Autodesk Inventor part; units mm, degrees
ref_plane "YZ Plane" through (0, 0, 0) normal (1, 0, 0) x (0, 1, 0)
ref_plane "XZ Plane" through (0, 0, 0) normal (0, 1, 0) x (-1, 0, 0)
ref_plane "XY Plane" through (0, 0, 0) normal (0, 0, 1) x (1, 0, 0)
sketch "Sketch1" plane through (0, 0, 0) normal (0, 1, 0) x (-1, 0, 0)
  line L0 (0, 0) -> (-101.6, 0)
  line L1 (-101.6, 0) -> (-101.6, -88.9)
  line L2 (-101.6, -88.9) -> (0, -88.9)
  line L3 (0, -88.9) -> (0, 0)
  line L4 (-50.8, -88.9) -> (-23.8125, -88.9)
  line L5 (-50.8, -88.9) -> (-77.7875, -88.9)
  line L6 (-77.7875, -88.9) -> (-77.7875, -82.55)
  line L7 (-23.8125, -88.9) -> (-23.8125, -82.55)
  circle A0 centre (-23.8125, -82.55) radius 1.905
  circle A1 centre (-77.7875, -82.55) radius 1.905
  dimension "d0" = 101.6
  dimension "d1" = 88.9
  dimension "d2" = 26.9875
  dimension "d3" = 26.9875
  dimension "d4" = 6.35
  dimension "d5" = 6.35
  dimension "d6" = 3.81
  dimension "d7" = 3.81
extrude "Extrusion1" add sketch "Sketch1" along normal blind 3.175
sketch "Sketch2" plane through (0, 0, 0) normal (0, -1, 0) x (1, 0, 0)
  line L0 (101.6, -88.9) -> (0, -88.9)
  line L1 (50.8, -88.9) -> (50.8, -12.7)
  line L2 (50.8, -12.7) -> (76.2, -12.7)
  line L3 (76.2, -12.7) -> (25.4, -12.7)
  line L4 (25.4, -12.7) -> (25.4, -6.35)
  line L5 (25.4, -6.35) -> (76.2, -6.35)
  line L6 (76.2, -6.35) -> (76.2, -12.7)
  point P0 (0, 0)
  dimension "d10" = 76.2
  dimension "d11" = 25.4
  dimension "d12" = 50.8
  dimension "d13" = 6.35
extrude "Extrusion2" add sketch "Sketch2" along normal blind 6.35
sketch "Sketch3" plane through (0, 3.175, 0) normal (0, 1, 0) x (1, 0, 0)
  line L0 (0, 0) -> (101.6, 0)
  line L1 (0, 0) -> (0, 34.29)
  line L2 (0, 88.9) -> (0, 0)
  line L3 (0, 34.29) -> (50.8, 34.29)
  line L4 (50.8, 34.29) -> (50.8, 40.64)
  line L5 (50.8, 40.64) -> (16.51, 40.64)
  line L6 (16.51, 40.64) -> (85.09, 40.64)
  line L7 (85.09, 40.64) -> (85.09, 27.94)
  line L8 (85.09, 27.94) -> (16.51, 27.94)
  line L9 (16.51, 27.94) -> (16.51, 40.64)
  dimension "d16" = 34.29
  dimension "d17" = 50.8
  dimension "d18" = 6.35
  dimension "d19" = 34.29
  dimension "d20" = 68.58
  dimension "d21" = 12.7
extrude "Extrusion3" add sketch "Sketch3" along normal blind 6.35
properties part number "mainboard"
Can you work these out from the model? Positions are in its coordinate system, mm. A direction names the side the tool comes from. Coordinates: 2 decimals unless noted, no trailing zeros. Loops run counter-clockwise (first coordinate to the right, second up) from the corner with the lowest first, then second, coordinate; pieces in that order, holes last. Notation, with made-up numbers: (57, 88) - (94, 88) arc R12 cw to (94, 107) - close; hole circle Ø1 at (78.25, 77). An arc over 180 degrees is marked (long way). Use a Markdown table: item, result.
Item 1: For faces 1 (the face through (76.2, -3, -9)), 2 (the face through (25.4, -3, -10)), 3 (the face through (51, -3, -12.7)), 4 (the face through (51, 6, -40.64)), 5 (the face through (50, -3, -6.35)), which set-ups out of +Z, -Z, +X, -X, +Y, -Y let a thin tool reach every point of the face, with its end or its side?
Numbers:
| item | result |
|---|---|
| face 1 | +Z, -Z, +X, -Y |
| face 2 | +Z, -Z, -X, -Y |
| face 3 | -Z, +X, -X, -Y |
| face 4 | -Z, +X, -X, +Y |
| face 5 | +Z, +X, -X, -Y |
Item 2: Will these pins go through, and if not, where does the flat tip stop? pin 1 (1.9 mm diameter, centred on x = 62, y = -4, fed in from -Z); pin 2 (3 mm diameter, centred on y = 5, z = -34.5, fed in from -X); pin 3 (7 mm diameter, centred on y = -4.5, z = -10.5, fed in from -X); pin 4 (8 mm diameter, centred on y = 5, z = -19, fed in from +X).
Numbers:
| item | result |
|---|---|
| pin 1 | stops at z = -12.7 |
| pin 2 | stops at x = 16.51 |
| pin 3 | stops at x = 25.4 |
| pin 4 | stops at x = 101.6 |
Item 3: I want a section at A-A on z = -82.55. Please give me the cut outline in (x, y) (1 decimal).
Numbers:
| item | result |
|---|---|
| outline | (0, 0) - (21.9, 0) - (21.9, 3.2) - (0, 3.2) - close; (25.7, 0) - (75.9, 0) - (75.9, 3.2) - (25.7, 3.2) - close; (79.7, 0) - (101.6, 0) - (101.6, 3.2) - (79.7, 3.2) - close |
Item 4: If I drill on probe 1 along X at (y, z) = (2.4, -82.55); probe 2 along Z at (x, y) = (33.5, 4.5); probe 3 along Y at (x, z) = (79.5, -74) (3 decimals), over which ranges is the centre line in solid material (lowest first)? Write a range as from..to.
Numbers:
| item | result |
|---|---|
| probe 1 | x = 0..21.91, 25.72..75.88, 79.69..101.6 |
| probe 2 | z = -40.64..-27.94 |
| probe 3 | y = 0..3.175 |
Item 5: I want a section at D-D on y = 5.75. Please give me the cut outline in (x, z).
Numbers:
| item | result |
|---|---|
| outline | (16.51, -40.64) - (85.09, -40.64) - (85.09, -27.94) - (16.51, -27.94) - close |
Item 6: I want a section at B-B on x = 77.5. Please give me the cut outline in (y, z) (3 decimals).
Numbers:
| item | result |
|---|---|
| outline | (0, -88.9) - (3.175, -88.9) - (3.175, -84.433) - (0, -84.433) - close; (0, -80.667) - (3.175, -80.667) - (3.175, -40.64) - (9.525, -40.64) - (9.525, -27.94) - (3.175, -27.94) - (3.175, 0) - (0, 0) - close |
Item 7: I want a section at C-C on z = -36. Please give me the cut outline in (x, y) (3 decimals), and give its area (3 significant figures).
Numbers:
| item | result |
|---|---|
| outline | (0, 0) - (101.6, 0) - (101.6, 3.175) - (85.09, 3.175) - (85.09, 9.525) - (16.51, 9.525) - (16.51, 3.175) - (0, 3.175) - close |
| area | 758 mm2 |
Item 8: We'd pull the mould along X, two halves only. Please class faces 6 (the face through (22.788, 1.565, -84.156)), 7 (the face through (52, 3.175, -44)), 8 (the face through (101.6, 2, -44)): released by +X, released by -X, zero draft, split by the parting line, or undercut.
Numbers:
| item | result |
|---|---|
| face 6 | undercut |
| face 7 | zero draft |
| face 8 | released by +X |
